from build123d import *

# Parameters (mm, degrees)
F1_DEPTH = 20


# Not quite as in the source:
# - a fillet or chamfer that OpenCascade refuses, or shapes differently, is made with other operations: its cross-section is extruded or revolved along the edge and cut away or added


with BuildPart() as f1:
    # F0 (on Front) → F1 (new body)
    with BuildSketch(Plane.XZ):
        with BuildLine():
            ThreePointArc((29.999922187, -0.0683284437), (29.9999805467, -0.034164244), (30, 0))
            ThreePointArc((30, 0), (21.2373474192, 21.189031941), (0.0683283603, 29.9999221872))
            Line((0.0683283603, 29.9999221872), (0.0683283603, 2.4316715563))
            ThreePointArc((0.0683283603, 2.4316715563), (1.8360953132, 1.6994385093), (2.5683283603, -0.0683284437))
            Line((2.5683283603, -0.0683284437), (29.999922187, -0.0683284437))
        make_face()
        with BuildLine():
            Line((24.9431081335, 2.4307376289), (9.7000780708, 2.4307376289))
            ThreePointArc((9.7000780708, 2.4307376289), (7.1211298187, 7.0206488379), (2.5683283603, 9.664558419))
            Line((2.5683283603, 9.664558419), (2.5683283603, 24.806357484))
            ThreePointArc((2.5683283603, 24.806357484), (17.7463297429, 17.6090092268), (24.9431081335, 2.4307376289))
        make_face(mode=Mode.SUBTRACT)
        with BuildLine():
            Line((0.0683283603, 2.4316715563), (0.0683283603, 29.9999221872))
            ThreePointArc((0.0683283603, 29.9999221872), (-21.2132034651, 21.2132034061), (-29.999922187, -0.0683284437))
            Line((-29.999922187, -0.0683284437), (-2.4316716397, -0.0683284437))
            ThreePointArc((-2.4316716397, -0.0683284437), (-1.7234334683, 1.675113425), (0, 2.4307376289))
            ThreePointArc((0, 2.4307376289), (0.034160989, 2.4314380635), (0.0683283603, 2.4316715563))
        make_face()
        with BuildLine():
            ThreePointArc((-24.8064514129, 2.4307376289), (-17.6096730223, 17.6090092268), (-2.4316716397, 24.806357484))
            Line((-2.4316716397, 24.806357484), (-2.4316716397, 9.6998439697))
            ThreePointArc((-2.4316716397, 9.6998439697), (-7.0714082408, 7.0707273665), (-9.7000780708, 2.4307376289))
            Line((-9.7000780708, 2.4307376289), (-24.8064514129, 2.4307376289))
        make_face(mode=Mode.SUBTRACT)
        with BuildLine():
            ThreePointArc((0.0683283603, -29.9999221872), (21.2132034061, -21.2132034651), (29.999922187, -0.0683284437))
            Line((29.999922187, -0.0683284437), (2.5683283603, -0.0683284437))
            ThreePointArc((2.5683283603, -0.0683284437), (1.8360953132, -1.8360953967), (0.0683283603, -2.5683284437))
            Line((0.0683283603, -2.5683284437), (0.0683283603, -29.9999221872))
        make_face()
        with BuildLine():
            ThreePointArc((24.9430142879, -2.5683284437), (17.7459978899, -17.7459979734), (2.5683283603, -24.9430143714))
            Line((2.5683283603, -24.9430143714), (2.5683283603, -9.664558419))
            ThreePointArc((2.5683283603, -9.664558419), (7.0710677813, -7.0710678424), (9.6645583968, -2.5683284437))
            Line((9.6645583968, -2.5683284437), (24.9430142879, -2.5683284437))
        make_face(mode=Mode.SUBTRACT)
        with BuildLine():
            Line((-2.4316716397, -0.0683284437), (-29.999922187, -0.0683284437))
            ThreePointArc((-29.999922187, -0.0683284437), (-21.1648329371, -21.2614638899), (0.0683283603, -29.9999221872))
            Line((0.0683283603, -29.9999221872), (0.0683283603, -2.5683284437))
            ThreePointArc((0.0683283603, -2.5683284437), (-1.6994385927, -1.8360953967), (-2.4316716397, -0.0683284437))
        make_face()
        with BuildLine():
            ThreePointArc((-2.4316716397, -24.9430143714), (-17.6093411694, -17.7459979734), (-24.8063575674, -2.5683284437))
            Line((-24.8063575674, -2.5683284437), (-9.6645583968, -2.5683284437))
            ThreePointArc((-9.6645583968, -2.5683284437), (-7.0209916464, -7.1207918311), (-2.4316716397, -9.6998439697))
            Line((-2.4316716397, -9.6998439697), (-2.4316716397, -24.9430143714))
        make_face(mode=Mode.SUBTRACT)
    extrude(amount=F1_DEPTH)

    # F2: fillet of radius 5 on 1 edges, made by hand

    # F2_s1 → F2_t2 (revolve, cut)
    with BuildSketch(Plane(origin=(0, 0, 0), x_dir=(0, 1, 0), z_dir=(-0.0022776148, 0, 0.9999974062))):
        with BuildLine():
            ThreePointArc((-15, 30), (-18.5355339059, 28.5355339059), (-20, 25))
            Line((-20, 25), (-20, 30))
            Line((-20, 30), (-15, 30))
        make_face()
    revolve(axis=Axis((0, -20, 0), (0, -1, 0)), mode=Mode.SUBTRACT)

    # F3: fillet of radius 5 on 1 edges, made by hand

    # F3_s1 → F3_t2 (revolve, cut)
    with BuildSketch(Plane(origin=(0, 0, 0), x_dir=(0, 1, 0), z_dir=(-0.0022776148, 0, 0.9999974062))):
        with BuildLine():
            ThreePointArc((0, 25), (-1.4644660941, 28.5355339059), (-5, 30))
            Line((-5, 30), (0, 30))
            Line((0, 30), (0, 25))
        make_face()
    revolve(axis=Axis((0, 0, 0), (0, -1, 0)), mode=Mode.SUBTRACT)


solid = f1.part
The listing builds one solid part. Answer for the finished solid, in the listing's coordinates (mm). A direction names the side the tool comes from. Give positions to 0.01 mm unless a question says otherwise; leave off trailing zeros. Order: outer loops, then holes, each group sorted by start corner. A loop starts at its lowest first (then second) coordinate and runs counter-clockwise, first axis right, second up. Notation, with made-up numbers: (-29, 65.5) - (2, 65.5) arc R6 ccw to (2, 74.5) - close; hole circle Ø1 at (62, 33). An arc over 180 degrees is marked (long way). Use one line per item in the form item = value.
1) Find section A-A on y = -10.75. Determine the outline of the cut face in (x, z), and give its area (3 significant figures).
Verdict:
outline = (30, -0.07) arc R30 ccw to (30, 0) arc R30 ccw (long way) to start; hole (-24.81, -2.57) arc R25 ccw to (-2.43, -24.94) - (-2.43, -9.7) arc R10 cw to (-9.66, -2.57) - close; hole (-24.81, 2.43) - (-9.7, 2.43) arc R10 cw to (-2.43, 9.7) - (-2.43, 24.81) arc R25 ccw to start; hole circle Ø5 at (0.07, -0.07); hole (2.57, -24.94) arc R25 ccw to (24.94, -2.57) - (9.66, -2.57) arc R10 cw to (2.57, -9.66) - close; hole (2.57, 9.66) arc R10 cw to (9.7, 2.43) - (24.94, 2.43) arc R25 ccw to (2.57, 24.81) - close
area = 1,460 mm^2
2) For faces 1 (the cylindrical face through (-7.07, -9.86, -7.07)), 2 (the flat face through (-2, -20, -2)), determine the directions among +Z, -Z, +X, -X, +Y, -Y from which every point of the face is accessible in a straight line to the end or side of a thin tool.
Verdict:
face_1 = +Y, -Y
face_2 = +Z, -Z, +X, -X, -Y
3) Each of these flat-tipped pins is pushed along its axis until it touches: pin 1 (10 mm diameter, centred on x = -18.5, y = -11, fed in from +Z); pin 2 (4.5 mm diameter, centred on y = -12, z = 15, fed in from +X); pin 3 (4 mm diameter, centred on y = -11.5, z = -5, fed in from +X). Where does it stop, or does it pass through?
Verdict:
pin_1 = 26.79
pin_2 = 27.16
pin_3 = 29.85
4) The mould has two halves that part along Z. Classify faces 3 (the cylindrical face through (7.02, -9.86, -7.12)), 4 (the flat face through (-2, 0, -2)): released by +Z, released by -Z, zero draft, split by the parting line, or undercut.
Verdict:
face_3 = undercut
face_4 = zero draft
5) Find section D-D on y = -3.25. Determine the outline of the cut face in (x, z), and give its area (3 significant figures).
Verdict:
outline = circle Ø59.37 at (0, 0); hole (-24.81, -2.57) arc R25 ccw to (-2.43, -24.94) - (-2.43, -9.7) arc R10 cw to (-9.66, -2.57) - close; hole (-24.81, 2.43) - (-9.7, 2.43) arc R10 cw to (-2.43, 9.7) - (-2.43, 24.81) arc R25 ccw to start; hole circle Ø5 at (0.07, -0.07); hole (2.57, -24.94) arc R25 ccw to (24.94, -2.57) - (9.66, -2.57) arc R10 cw to (2.57, -9.66) - close; hole (2.57, 9.66) arc R10 cw to (9.7, 2.43) - (24.94, 2.43) arc R25 ccw to (2.57, 24.81) - close
area = 1,400 mm^2
6) Find section B-B on x = 16.5. Give the number of separate pieces and of enclosed holes in the cut face, and give its area (3 significant figures).
Verdict:
separate_pieces = 3
enclosed_holes = 0
area = 322 mm^2
7) Consider probe 1 along Z at (x, y) = (20, -3.25); probe 2 along X at (y, z) = (-12.5, -13); probe 3 along Z at (x, y) = (-11, -10). Determine where each line is inside the solid, lowest interval first. Write a range as [from, to].
Verdict:
probe_1 = [-21.93, -15.16], [-2.57, 2.43], [15.02, 21.93]
probe_2 = [-27.04, -21.33], [-2.43, 2.57], [21.46, 27.04]
probe_3 = [-27.91, -22.48], [-2.57, 2.43], [22.35, 27.91]
